from build123d import *

# Parameters (mm, degrees)
F0_R     = 209.55
F0_R_2   = 15.875
F0_R_3   = 101.6
F1_DEPTH = 55.626
F2_R     = 130.175
F2_R_2   = 101.6
F3_DEPTH = 6.35
F4_R     = 2.54


with BuildPart() as f1:
    # F0 (on Front) → F1 (new body)
    with BuildSketch(Plane.XZ):
        Circle(F0_R)
        with Locations((-123.478522, -123.478522)):
            Circle(F0_R_2, mode=Mode.SUBTRACT)
        with Locations((-45.196276, -168.674797)):
            Circle(F0_R_2, mode=Mode.SUBTRACT)
        with Locations((-168.674797, -45.196276)):
            Circle(F0_R_2, mode=Mode.SUBTRACT)
        with Locations((45.196276, -168.674797)):
            Circle(F0_R_2, mode=Mode.SUBTRACT)
        with Locations((123.478522, -123.478522)):
            Circle(F0_R_2, mode=Mode.SUBTRACT)
        with Locations((168.674797, -45.196276)):
            Circle(F0_R_2, mode=Mode.SUBTRACT)
        with Locations((-168.674797, 45.196276)):
            Circle(F0_R_2, mode=Mode.SUBTRACT)
        with Locations((-123.478522, 123.478522)):
            Circle(F0_R_2, mode=Mode.SUBTRACT)
        with Locations((-45.196276, 168.674797)):
            Circle(F0_R_2, mode=Mode.SUBTRACT)
        Circle(F0_R_3, mode=Mode.SUBTRACT)
        with Locations((168.674797, 45.196276)):
            Circle(F0_R_2, mode=Mode.SUBTRACT)
        with Locations((45.196276, 168.674797)):
            Circle(F0_R_2, mode=Mode.SUBTRACT)
        with Locations((123.478522, 123.478522)):
            Circle(F0_R_2, mode=Mode.SUBTRACT)
    extrude(amount=F1_DEPTH)

    # F2 (on face) → F3 (join)
    with BuildSketch(Plane.XZ.offset(55.626)):
        Circle(F2_R)
        Circle(F2_R_2, mode=Mode.SUBTRACT)
    extrude(amount=F3_DEPTH)

    # F4
    f4_edges = [f1.edges().sort_by_distance(p)[0] for p in [
        (-209.55, -55.626, 0),
        (-209.55, 0, 0),
        (-130.175, -61.976, 0),
        (-130.175, -55.626, 0),
    ]]
    fillet(f4_edges, radius=F4_R)


solid = f1.part
Model file for the job. Use its own axes, mm. Give positions to 0.01 mm unless a question says otherwise; leave off trailing zeros. Write each loop counter-clockwise with the first axis right and the second up, starting at its lowest first coordinate (ties: lowest second). Pieces come first, ordered by that corner, then holes. Notation, with made-up numbers: M 33,67.5 L 92,67.5 A21 cw 92,76.5 Z; hole C -32,74 d3. An arc over 180 degrees is marked long. One line per item, written item: value. Start each with the question number.
Q1. Saw through at A-A, the plane x = 0. Write the cut outline in (y, z) (3 decimals).
Q2. Saw through at C-C, the plane y = -40.5. State how many separate pieces and enclosed holes the cut face has, plus the area to 3 significant figures.
Q3. Saw through at B-B, the plane z = 0. Write the cut outline in (x, y) (3 decimals), plus the area to 3 significant figures.
Q4. Two-plate mould, pull along Z, no slides. Class faces 1 (the cylindrical face through (-47.263, -27.424, -152.935)), 2 (the flat face through (-95, -55.626, 95)), 3 (the cylindrical face through (-103.3, -58.79, -79.21)): +Z half, -Z half, draft (parallel to the pull), parting line (faces both ways), or undercut.
Q5. Drop flat-ended pins along their axis: pin 1 Ø3 at (y, z) = (-44.5, -103.5) entering from +X; pin 2 Ø10 at (y, z) = (-20.5, 164) entering from -X; pin 3 Ø1.5 at (x, y) = (-46.5, -8.5) entering from -Z. Give the stop position or say it passes through.
Q6. Probe probe 1 along Z at (x, y) = (42.5, -20); probe 2 along Z at (x, y) = (115, -46); probe 3 along X at (y, z) = (-13.5, -161). List the from-to ranges inside material, lowest first. Write a range as [from, to].
Output values:
1. outline: M -61.976,-127.635 A2.54 ccw -59.436,-130.175 L -58.166,-130.175 A2.54 cw -55.626,-132.715 L -55.626,-207.01 A2.54 ccw -53.086,-209.55 L -2.54,-209.55 A2.54 ccw 0,-207.01 L 0,-101.6 L -61.976,-101.6 Z; M -61.976,101.6 L 0,101.6 L 0,207.01 A2.54 ccw -2.54,209.55 L -53.086,209.55 A2.54 ccw -55.626,207.01 L -55.626,132.715 A2.54 cw -58.166,130.175 L -59.436,130.175 A2.54 ccw -61.976,127.635 Z
2. separate pieces: 1
2. enclosed holes: 13
2. area: 96,000 mm²
3. outline: M -209.55,-53.086 A2.54 ccw -207.01,-55.626 L -132.715,-55.626 A2.54 cw -130.175,-58.166 L -130.175,-59.436 A2.54 ccw -127.635,-61.976 L -101.6,-61.976 L -101.6,0 L -207.01,0 A2.54 ccw -209.55,-2.54 Z; M 101.6,-61.976 L 127.635,-61.976 A2.54 ccw 130.175,-59.436 L 130.175,-58.166 A2.54 cw 132.715,-55.626 L 207.01,-55.626 A2.54 ccw 209.55,-53.086 L 209.55,-2.54 A2.54 ccw 207.01,0 L 101.6,0 Z
3. area: 12,400 mm²
4. face 1: undercut
4. face 2: draft
4. face 3: parting line
5. pin 1: stops at x = 183.05
5. pin 2: stops at x = -136.49
5. pin 3: stops at z = -204.49
6. probe 1: z = [-205.19, -184.32], [-153.03, -92.28], [92.28, 153.03], [184.32, 205.19]
6. probe 2: z = [-175.17, -136.9], [-110.06, 110.06], [136.9, 175.17]
6. probe 3: x = [-134.13, -59.09], [-31.3, 31.3], [59.09, 134.13]
